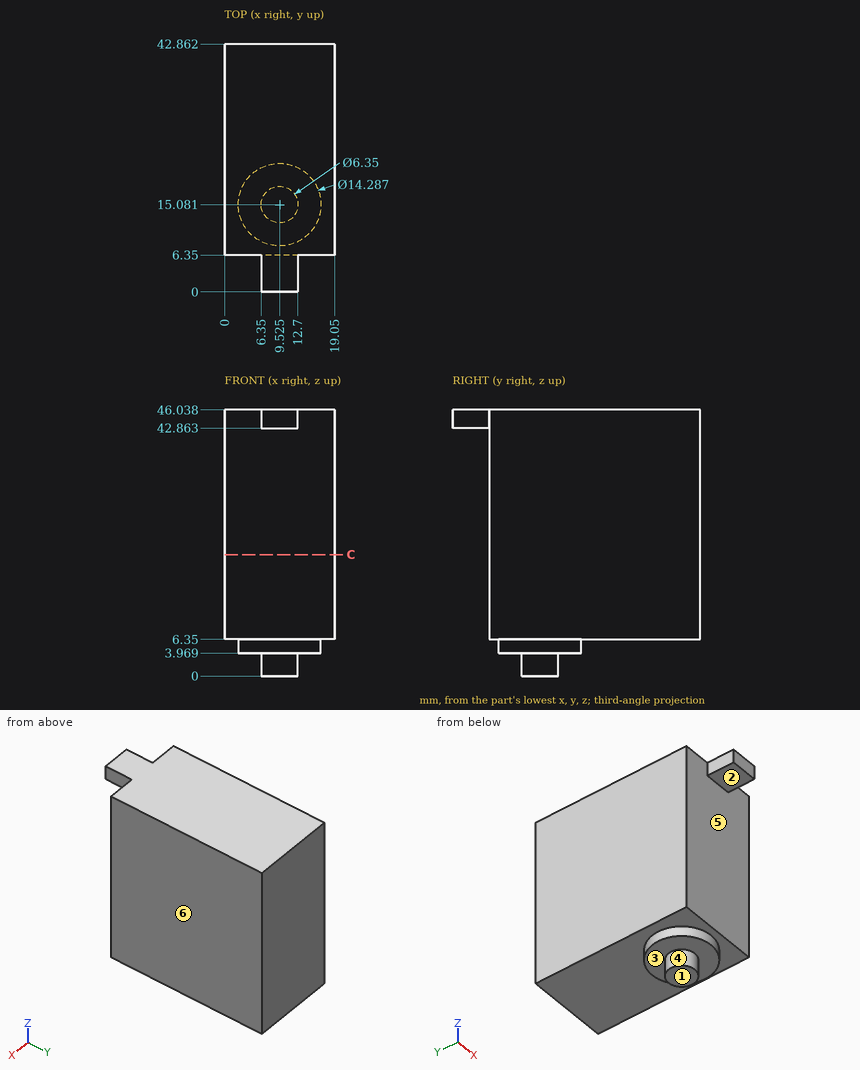
Here's the drawing with two shaded views (mm, measured from the low corner). I have some questions. A direction names the side the tool comes from. Give positions to 0.01 mm unless a question says otherwise; leave off trailing zeros. Loops run counter-clockwise (first coordinate to the right, second up) from the corner with the lowest first, then second, coordinate; pieces in that order, holes last. Notation, with made-up numbers: M 1,-37 L 27,-37 A29 ccw 27,-16 Z; hole C 42,-22 d3. An arc over 180 degrees is marked long. One line per item, written item: value. Start each with the question number.
1) I'm going to push flat-ended pins straight in: pin 1 (2.5 mm diameter, centred on y = 2, z = 44, fed in from +X); pin 2 (6 mm diameter, centred on x = 7.5, z = 36, fed in from -Y); pin 3 (1.9 mm diameter, centred on x = 11, y = 4, fed in from -Z). Where does each tip first touch, or does it pass through?
2) If we section it at C-C, the plane z = 21: Write out the boundary of the cut face in (x, y).
3) On a 3-axis mill with a long thin cutter (end or side, diameter ignored), from which of +Z, -Z, +X, -X, +Y, -Y can I reach the whole of each face in a straight line? I mean the marked faces 1, 2 and 3. Say none if no direction works.
4) Thinking about a two-plate mould opening in X: for the marked faces 4, 5 and 6, which applies, +X half, -X half, draft (parallel to the pull), parting line (faces both ways), or undercut?
5) If I drill on line 1 (Y direction, x = 4.5, z = 8); line 2 (Z direction, x = 6.75, y = 32); line 3 (Z direction, x = 5.25, y = 12.5), over which ranges is the centre line in solid material (lowest first)? Write a range as [from, to].
Completed:
1. pin 1: stops at x = 12.7
1. pin 2: stops at y = 6.35
1. pin 3: stops at z = 42.86
2. outline: M 0,6.35 L 19.05,6.35 L 19.05,42.86 L 0,42.86 Z
3. face 1: -Z, +X, -X, +Y, -Y
3. face 2: -Z, +X, -X, -Y
3. face 3: -Z
4. face 4: parting line
4. face 5: draft
4. face 6: +X half
5. line 1: y = [6.35, 42.86]
5. line 2: z = [6.35, 46.04]
5. line 3: z = [3.97, 46.04]
